Model file for the job. Use its own axes, mm. A direction names the side the tool comes from. Coordinates: 2 decimals unless noted, no trailing zeros. Order: outer loops, then holes, each group sorted by start corner. A loop starts at its lowest first (then second) coordinate and runs counter-clockwise, first axis right, second up. Notation, with made-up numbers: (53.25, 3.5) -> (78.25, 3.5) arc R17 cw to (78.25, 18.5) -> close; hole circle Ø3 at (-16, 8). An arc over 180 degrees is marked (long way). Use CSV: the item, a comma, the result in double quotes. Start each with the question number.
(1) Cut at C-C on z = -2.5. Write the cut outline in (x, y).
(2) Cut at A-A on x = 22.5. Write the cut outline in (y, z), plus the area to 3 significant figures.
(3) Cut at B-B on z = 9. Write the cut outline in (x, y), plus the area to 3 significant figures.
(4) Cut at D-D on y = 24. Write the cut outline in (x, z), plus the area to 3 significant figures.
(5) Tool access for faces 4 (the flat face through (18.6, 2.8, 0)), 5 (the flat face through (-8, 11, 11)), 6 (the flat face through (9.7, 1, 20.3)), 7 (the flat face through (0, -12, -4)), 8 (the cylindrical face through (-9.89, 10.51, 17.99)): list every direction of +Z, -Z, +X, -X, +Y, -Y with a clear straight run to the whole face (end or side of a thin tool).
(6) Probe L1, parallel to X at y = 5.5, z = 19; L2, parallel to X at y = 5.5, z = 10; L3, parallel to Y at x = -22.5, z = -1.5. List the from-to ranges inside material, lowest first.
(7) Pin check, flat tips, straight feed: pin 1 Ø2 at (y, z) = (10.5, 17) entering from -X; pin 2 Ø8.5 at (x, y) = (-22, 1.5) entering from +Z; pin 3 Ø3 at (x, z) = (-12, 17.5) entering from -Y; pin 4 Ø7 at (x, y) = (-22.5, 0) entering from -Z. Stop position of each tip, or through.
(8) Pull direction X, two halves, no side cores. Call faces 1 (the flat face through (-14, 11, 11)), 2 (the cylindrical face through (-11, 32, 25)), 3 (the cylindrical face through (18, 0, -4)): pulls with the +X half, pulls with the -X half, needs draft (parallel to the pull), parting line crosses it, or undercut.
Autodesk Fusion 360 part; units mm, degrees
sketch "草图1" plane through (0, 0, 0) normal (0, 0, 1) x (1, 0, 0)
  line L0 (-31, 12) -> (31, 12)
  line L1 (31, 12) -> (31, -12)
  line L2 (31, -12) -> (-31, -12)
  line L3 (-31, -12) -> (-31, 12)
  circle A0 centre (-22.5, 0) radius 4.5
  circle A1 centre (22.5, 0) radius 4.5
  line L4 (0, 20) -> (0, -25) construction
  line L5 (35, 0) -> (-34, 0) construction
  dimension "d1" = 24
  dimension "d2" = 62
  dimension "d3" = 9
  dimension "d4" = 45
extrude "拉伸1" add sketch "草图1" against normal blind 8 makes body 1
ref_plane "工作平面1" through (-14, 0, -4) normal (-1, 0, 0) x (0, 1, 0)
sketch "草图2" plane through (-14, 0, 0) normal (-1, 0, 0) x (0, -1, 0)
  line L0 (-12, 0) -> (12, 0)
  line L1 (12, 0) -> (12, 6)
  line L2 (12, 6) -> (-18.2642, 27.1915)
  line L3 (-12, 0) -> (-29.1954, 10.4555)
  arc A0 (-18.2642, 27.1915) -> (-29.1954, 10.4555) centre (-24, 19) ccw
  circle A1 centre (-24, 19) radius 4
  line L4 (0, 23) -> (0, -19) construction
  line L5 (12, -8) -> (-12, -8) construction
  line L6 (12, 0) -> (12, -8) construction
  dimension "d8" = 6
  dimension "d9" = 27
  dimension "d10" = 36
  dimension "d11" = 8
  dimension "d12" = 10
  dimension "d13" = 24
extrude "拉伸2" add sketch "草图2" against normal blind 6 separate body makes body 2
ref_plane "工作平面2" through (-11, 1, 3) normal (0, -1, 0) x (0, 0, -1)
sketch "草图3" plane through (0, 1, 0) normal (0, -1, 0) x (-1, 0, 0)
  circle A0 centre (11, -19) radius 3
  circle A1 centre (11, -19) radius 1.5
  line L0 (-31, 8) -> (31, 8)
  line L1 (8, -27.1915) -> (8, -6)
  dimension "d17" = 6
  dimension "d18" = 3
  dimension "d19" = 27
  dimension "d20" = 3
extrude "拉伸3" add sketch "草图3" along normal up to surface end surface at (-10, 20.005, 18.8006) on bodies 2 bodies 2
extrude "拉伸4" cut sketch "草图3" along normal up to surface contours A1 end surface at (-10, 20.005, 18.8006) on bodies 2 bodies 2
copy_body "复制和粘贴实体1" bodies 2 makes body 3
move_body "移动1" bodies 3 to x (1, 0, 0) y (0, 1, 0) z (0, 0, 1) at (22, 0, 0)
combine "合并1" operation add target body 1 tool bodies 3 2
Outcome:
1,outline,"(-31, -12) -> (31, -12) -> (31, 12) -> (-31, 12) -> close; hole circle Ø9 at (-22.5, 0); hole circle Ø9 at (22.5, 0)"
2,outline,"(-12, -8) -> (-4.5, -8) -> (-4.5, 0) -> (-12, 0) -> close; (4.5, -8) -> (12, -8) -> (12, 0) -> (4.5, 0) -> close"
2,area,"120 mm2"
3,outline,"(-14, -7.72) -> (-8, -7.72) -> (-8, 26.8) -> (-14, 26.8) -> close; (8, -7.72) -> (14, -7.72) -> (14, 26.8) -> (8, 26.8) -> close"
3,area,"414 mm2"
4,outline,"(-14, 7.3) -> (-8, 7.3) -> (-8, 15) -> (-14, 15) -> close; (-14, 23) -> (-8, 23) -> (-8, 29) -> (-14, 29) -> close; (8, 7.3) -> (14, 7.3) -> (14, 15) -> (8, 15) -> close; (8, 23) -> (14, 23) -> (14, 29) -> (8, 29) -> close"
4,area,"164 mm2"
5,face 4,"+Z, +X, +Y, -Y"
5,face 5,"+Z, +Y, -Y"
5,face 6,"+Z, +X, -X, -Y"
5,face 7,"+Z, -Z, +X, -X, -Y"
5,face 8,"-Y"
6,L1,"-14 to -12.5, -9.5 to -8, 8 to 9.5, 12.5 to 14"
6,L2,"-14 to -8, 8 to 14"
6,L3,"-12 to -4.5, 4.5 to 12"
7,pin 1,"x = -14"
7,pin 2,"z = 0"
7,pin 3,"y = 1"
7,pin 4,"through"
8,face 1,"pulls with the -X half"
8,face 2,"needs draft"
8,face 3,"undercut"
